Drawing for the job (mm, zero at the part's lowest x, y, z). A direction names the side the tool comes from. Round coordinates to 2 decimals unless told otherwise and drop trailing zeros. Order: outer loops, then holes, each group sorted by start corner. A loop starts at its lowest first (then second) coordinate and runs counter-clockwise, first axis right, second up. Notation, with made-up numbers: (84.25, 49.5) - (104.25, 49.5) arc R25 cw to (104.25, 86.5) - close; hole circle Ø9 at (37, 8). An arc over 180 degrees is marked (long way). Put each result on its own line as item: value. Start each with the question number.
Item 1: Saw through at B-B on x = 10. List the corners of the cut face in (y, z).
Item 2: Probe probe 1 along X at (y, z) = (2.75, 6.5) (1 decimal); probe 2 along Z at (x, y) = (6.25, 5.75) (1 decimal); probe 3 along Z at (x, y) = (9, 2) (1 decimal). List the from-to ranges inside material, lowest first.
Item 3: Which spindle directions (+Z, -Z, +X, -X, +Y, -Y) get a long thin tool onto all of the face, cutting with end or side? Do the marked faces 4 and 5. Say none if no direction does.
Item 4: Mould opens along X. For the marked faces 1, 2 and 3 say: pulls with the +X half, pulls with the -X half, needs draft (parallel to the pull), parting line crosses it, or undercut.
Item 5: Saw through at A-A on z = 6.35. List the corners of the cut face in (x, y).
Item 6: Pin check, flat tips, straight feed: pin 1 Ø7 at (x, z) = (7.94, 6.35) entering from +Y; pin 2 Ø0.6 at (x, y) = (3.5, 3) entering from -Z (1 decimal); pin 3 Ø2 at (x, y) = (2, 3.5) entering from -Z (1 decimal); pin 4 Ø1 at (x, y) = (11, 1) entering from +Z (1 decimal). Stop position of each tip, or through.
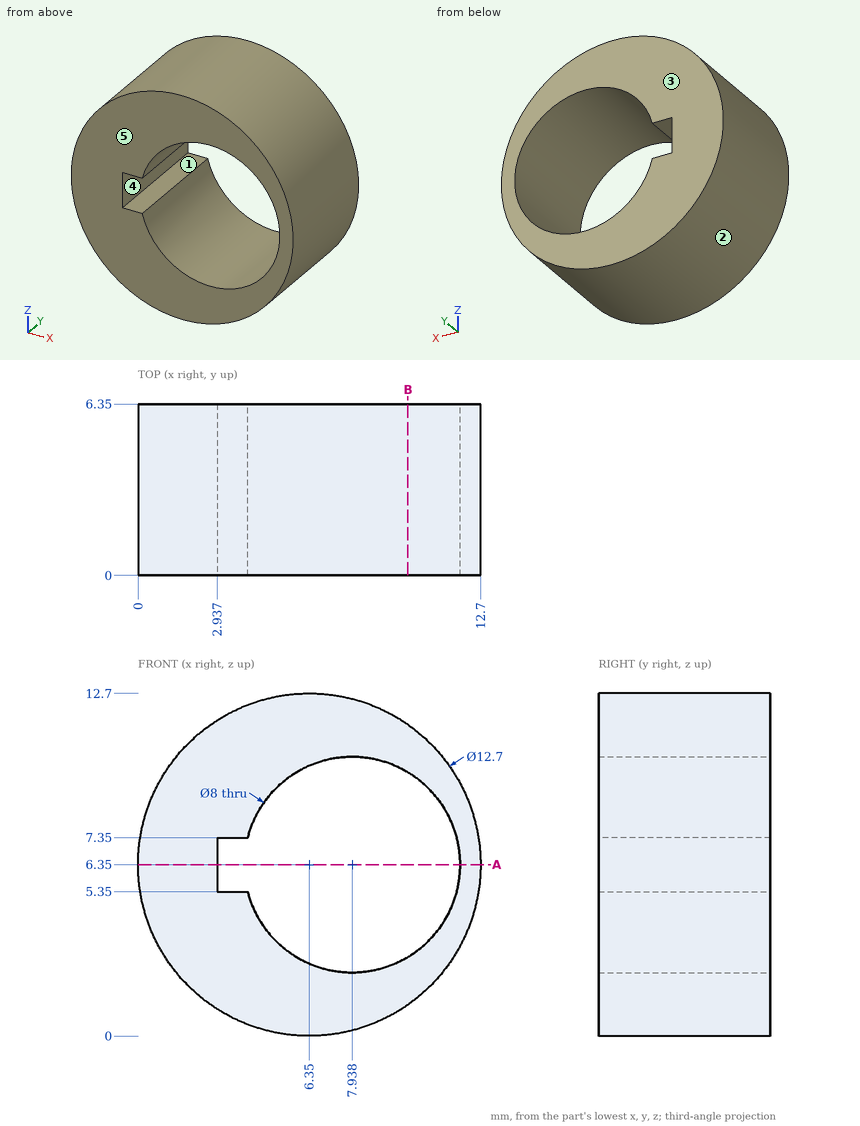
Results found:
1. outline: (0, 1.15) - (6.35, 1.15) - (6.35, 2.92) - (0, 2.92) - close; (0, 9.78) - (6.35, 9.78) - (6.35, 11.55) - (0, 11.55) - close
2. probe 1: x = 0 to 2.9, 11.9 to 12.7
2. probe 2: z = 0 to 2.7, 10 to 12.7
2. probe 3: z = 0.6 to 2.5, 10.2 to 12.1
3. face 4: +Y, -Y
3. face 5: +Z, -Z, +X, -X, -Y
4. face 1: undercut
4. face 2: parting line crosses it
4. face 3: needs draft
5. outline: (0, 0) - (2.94, 0) - (2.94, 6.35) - (0, 6.35) - close; (11.94, 0) - (12.7, 0) - (12.7, 6.35) - (11.94, 6.35) - close
6. pin 1: passes through
6. pin 2: stops at z = 0.5
6. pin 3: stops at z = 1
6. pin 4: stops at z = 11.2
